The figure shows three views and two pictorial views of one solid part (mm, origin at its lowest corner). Answer the questions. A direction names the side the tool comes from. Give positions to 0.01 mm unless a question says otherwise; leave off trailing zeros. Write each question's results on one line, items separated by ' | '. Start each with the question number.
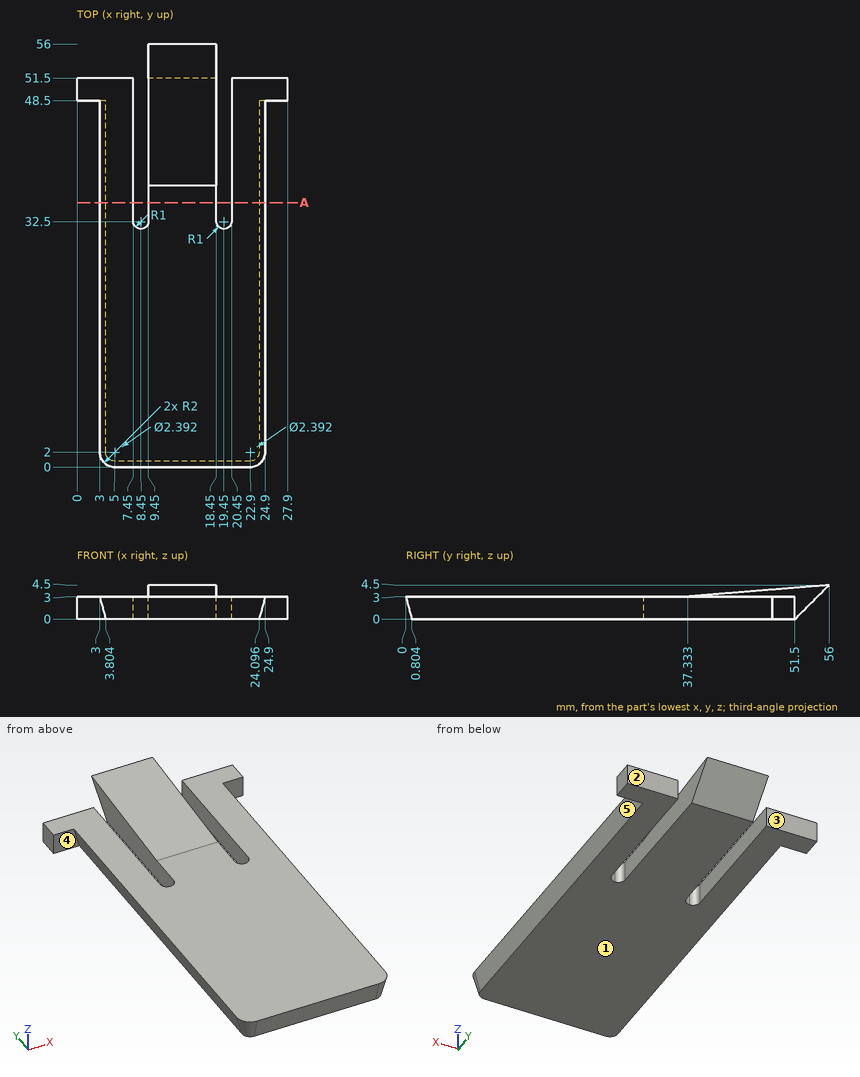
Q1. A cutting plane is placed at A-A, the plane y = 35. Give the number of separate pieces and of enclosed holes in the cut face, and give its area (3 significant figures).
Q2. Given pin 1 (1 mm diameter, centred on x = 11.5, z = 1.5, fed in from -Y); pin 2 (0.9 mm diameter, centred on y = 39, z = 1, fed in from -X) (1 decimal); pin 3 (2.5 mm diameter, centred on x = 26, z = 2, fed in from -Y), each flat-ended and moving along its own axis, determine where each tip first touches the part or whether it passes through.
Q3. A tool of negligible diameter and unlimited length cuts with its end or side. For the marked faces 1, 2, 3, 4 and 5, from which of +Z, -Z, +X, -X, +Y, -Y can it reach the whole face along a straight path? Write none if from no direction.
Q4. Consider L1, parallel to X at y = 34, z = 1.85; L2, parallel to Z at x = 10.25, y = 12.5; L3, parallel to Y at x = 2.75, z = 0.95. Determine where each line is inside the solid, lowest interval first.
Result:
1) separate pieces: 3 | enclosed holes: 0 | area: 51.3 mm2
2) pin 1: stops at y = 0.27 | pin 2: stops at x = 3.4 | pin 3: stops at y = 48.5
3) face 1: -Z, +X, -X, +Y, -Y | face 2: +Z, -Z, +X, +Y | face 3: +Z, -Z, -X, +Y | face 4: -Z, -X, -Y | face 5: -Z, +X, -Y
4) L1: x = 3.31 to 7.45, 9.45 to 18.45, 20.45 to 24.59 | L2: z = 0 to 3 | L3: y = 48.5 to 51.5
